```python
from build123d import *

# Parameters (mm, degrees)
CYLINDER032_R     = 1.5
CYLINDER032_DEPTH = 5.2
CYLINDER026_R     = 1.2
CYLINDER026_DEPTH = 4.8
CYLINDER028_R     = 1.2
CYLINDER028_DEPTH = 4.8
CYLINDER024_R     = 1.2
CYLINDER024_DEPTH = 4.8
CYLINDER031_R     = 1.2
CYLINDER031_DEPTH = 4.8
CYLINDER023_R     = 10.5
CYLINDER023_DEPTH = 5
CYLINDER022_R     = 12
CYLINDER022_DEPTH = 6


with BuildPart() as cylinder032:
    # Cylinder032 → Cylinder032 (new body)
    with BuildSketch(Plane(origin=(10, 0, 4.3), x_dir=(1, 0, 0), z_dir=(0, 0, 1))):
        Circle(CYLINDER032_R)
    extrude(amount=CYLINDER032_DEPTH)


with BuildPart() as cylinder026:
    # Cylinder026 → Cylinder026 (new body)
    with BuildSketch(Plane(origin=(0, -6.8, -1), x_dir=(1, 0, 0), z_dir=(0, 0, 1))):
        Circle(CYLINDER026_R)
    extrude(amount=CYLINDER026_DEPTH)


with BuildPart() as cylinder028:
    # Cylinder028 → Cylinder028 (new body)
    with BuildSketch(Plane(origin=(6.303301, -0.003301, -1), x_dir=(1, 0, 0), z_dir=(0, 0, 1))):
        Circle(CYLINDER028_R)
    extrude(amount=CYLINDER028_DEPTH)


with BuildPart() as cylinder024:
    # Cylinder024 → Cylinder024 (new body)
    with BuildSketch(Plane(origin=(0, 6.3, -1), x_dir=(1, 0, 0), z_dir=(0, 0, 1))):
        Circle(CYLINDER024_R)
    extrude(amount=CYLINDER024_DEPTH)


with BuildPart() as cylinder031:
    # Cylinder031 → Cylinder031 (new body)
    with BuildSketch(Plane(origin=(-6.296699, -0.003301, -1), x_dir=(1, 0, 0), z_dir=(0, 0, 1))):
        Circle(CYLINDER031_R)
    extrude(amount=CYLINDER031_DEPTH)


with BuildPart() as cylinder023:
    # Cylinder023 → Cylinder023 (new body)
    with BuildSketch(Plane.XY.offset(-1.5)):
        Circle(CYLINDER023_R)
    extrude(amount=CYLINDER023_DEPTH)


with BuildPart() as fusion008:
    # Cylinder022 → Cylinder022 (new body)
    with BuildSketch(Plane.XY.offset(-1.45)):
        Circle(CYLINDER022_R)
    extrude(amount=CYLINDER022_DEPTH)

    # Cut014: cut Cylinder023
    add(cylinder023.part, mode=Mode.SUBTRACT)

    # Fusion007: union Cylinder026, Cylinder028, Cylinder024, Cylinder031
    add(cylinder026.part)
    add(cylinder028.part)
    add(cylinder024.part)
    add(cylinder031.part)

    # Fusion008: union Cylinder032
    add(cylinder032.part)


solid = fusion008.part
```
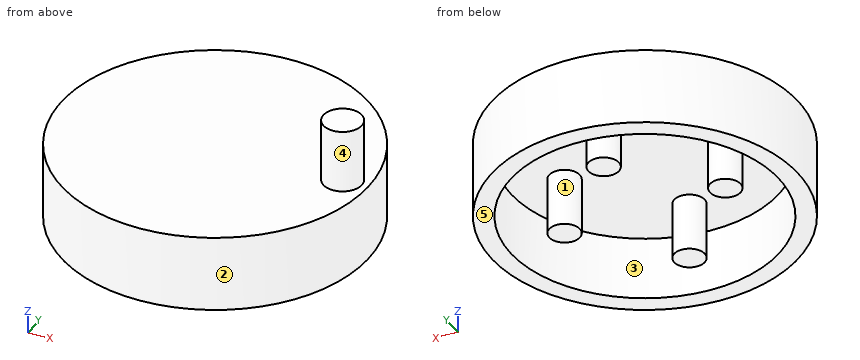
Geometry: final body of the model. Coordinates: model frame, mm. Face numbers are marked on the shaded views. A direction names the side the tool comes from. Give positions to 0.01 mm unless a question says otherwise; leave off trailing zeros. Loops run counter-clockwise (first coordinate to the right, second up) from the corner with the lowest first, then second, coordinate; pieces in that order, holes last. Notation, with made-up numbers: (-22, -21.5) -> (-6, -21.5) arc R28 ccw to (-6, 3.5) -> close; hole circle Ø6 at (71, -21). An arc over 180 degrees is marked (long way). Use one line per item in the form item = value.
Item 1: Pin query (flat end, axial travel): P1, Ø6, axis at y = 6.5, z = 5.5, coming from the -X side; P2, Ø5, axis at x = 5.5, y = -6, coming from the +Z side; P3, Ø1.9, axis at x = 6.5, y = 0.5, coming from the -Z side; P4, Ø1.5, axis at x = 4.5, z = 7, coming from the +Y side. Return the tip coordinate at first contact, or that it passes through.
A:
P1 = -11.43
P2 = 4.55
P3 = -1
P4 = through
Item 2: Section query B-B on z = 0. Output: boundary loops of the cut face in (x, y).
A:
outline = circle Ø24 at (0, 0); circle Ø2.4 at (-6.3, 0); circle Ø2.4 at (0, -6.8); circle Ø2.4 at (0, 6.3); circle Ø2.4 at (6.3, 0); hole circle Ø21 at (0, 0)
Item 3: Section query C-C on y = 6.3. Output: boundary loops of the cut face in (x, z), and give its area (3 significant figures).
A:
outline = (-10.21, -1.45) -> (-8.4, -1.45) -> (-8.4, 3.5) -> (-1.2, 3.5) -> (-1.2, -1) -> (1.2, -1) -> (1.2, 3.5) -> (8.4, 3.5) -> (8.4, -1.45) -> (10.21, -1.45) -> (10.21, 4.55) -> (-10.21, 4.55) -> close
area = 50.2 mm^2
Item 4: Line query: probe 1 along Y at (x, z) = (0, 0.1); probe 2 along Y at (x, z) = (-0.75, 3); probe 3 along X at (y, z) = (-7.5, 3.25). Output: solid intervals per line, ascending.
A:
probe_1 = -12 to -10.5, -8 to -5.6, 5.1 to 7.5, 10.5 to 12
probe_2 = -11.98 to -10.47, -7.74 to -5.86, 5.36 to 7.24, 10.47 to 11.98
probe_3 = -9.37 to -7.35, -0.97 to 0.97, 7.35 to 9.37
Item 5: Draft query along X for the marked faces 3, 4 and 5. Return one class per face: pulls with the +X half, pulls with the -X half, needs draft (parallel to the pull), parting line crosses it, or undercut.
A:
face_3 = undercut
face_4 = parting line crosses it
face_5 = needs draft
Item 6: Section query A-A on x = 0. Output: boundary loops of the cut face in (y, z).
A:
outline = (-12, -1.45) -> (-10.5, -1.45) -> (-10.5, 3.5) -> (-8, 3.5) -> (-8, -1) -> (-5.6, -1) -> (-5.6, 3.5) -> (5.1, 3.5) -> (5.1, -1) -> (7.5, -1) -> (7.5, 3.5) -> (10.5, 3.5) -> (10.5, -1.45) -> (12, -1.45) -> (12, 4.55) -> (-12, 4.55) -> close
Item 7: Access query for the marked faces 1 and 2. Directions: +Z, -Z, +X, -X, +Y, -Y. A direction counts if a zero-diameter tool reaches every point of the face in a straight line with its end or side. Return the directions, or none.
A:
face_1 = -Z
face_2 = +Z, -Z
Item 8: Section query D-D on x = -8.5. Output: boundary loops of the cut face in (y, z).
A:
outline = (-8.47, -1.45) -> (-6.16, -1.45) -> (-6.16, 3.5) -> (6.16, 3.5) -> (6.16, -1.45) -> (8.47, -1.45) -> (8.47, 4.55) -> (-8.47, 4.55) -> close
